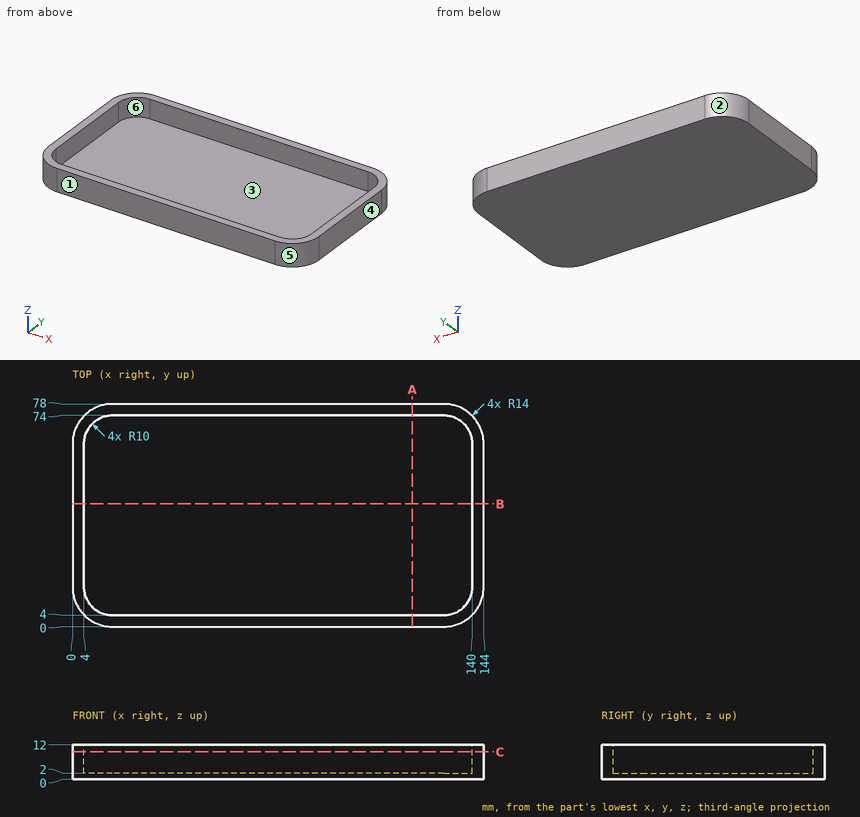
Geometry check sheet. Reference: drawing and pictorial views, mm from the part's lowest x, y, z. A direction names the side the tool comes from. Coordinates: 2 decimals unless noted, no trailing zeros. Write each loop counter-clockwise with the first axis right and the second up, starting at its lowest first coordinate (ties: lowest second). Pieces come first, ordered by that corner, then holes.
Item 1: Depth check by flat-ended pin: pin 1 Ø1 at (x, y) = (117, 37.5) entering from +Z. Enter the tip coordinate at first touch or a pass-through.
Numbers:
pin 1: stops at z = 2
Item 2: Scan lines: probe 1 along Y at (x, z) = (126.5, 3.75); probe 2 along X at (y, z) = (48, 11.25); probe 3 along Z at (x, y) = (51.5, 39.5). Record each from-to range of solid material in increasing order.
Numbers:
probe 1: y = 0 to 4, 74 to 78
probe 2: x = 0 to 4, 140 to 144
probe 3: z = 0 to 2
Item 3: Cross-section at C-C on z = 9.5. Record the boundary of the cut face in (x, y), then the cut area to 3 significant figures.
Numbers:
outline: (0, 14) arc R14 ccw to (14, 0) - (130, 0) arc R14 ccw to (144, 14) - (144, 64) arc R14 ccw to (130, 78) - (14, 78) arc R14 ccw to (0, 64) - close; hole (4, 14) arc R10 ccw to (14, 4) - (130, 4) arc R10 ccw to (140, 14) - (140, 64) arc R10 ccw to (130, 74) - (14, 74) arc R10 ccw to (4, 64) - close
area: 1,630 mm2
Item 4: Mould release check, pull along X, two halves, no side actions. Record for the marked faces 1, 2, 3 and 4: released by +X, released by -X, zero draft, split by the parting line, or undercut.
Numbers:
face 1: zero draft
face 2: released by -X
face 3: undercut
face 4: released by +X
Item 5: Cross-section at A-A on x = 119. Record the boundary of the cut face in (y, z).
Numbers:
outline: (0, 0) - (78, 0) - (78, 12) - (74, 12) - (74, 2) - (4, 2) - (4, 12) - (0, 12) - close
Item 6: Access from +Z, -Z, +X, -X, +Y, -Y to the whole of each face (thin tool, end or side, straight path). Record for the marked faces 5 and 6.
Numbers:
face 5: +Z, -Z, +X, -Y
face 6: +Z
Item 7: Cross-section at B-B on y = 43. Record the boundary of the cut face in (x, z).
Numbers:
outline: (0, 0) - (144, 0) - (144, 12) - (140, 12) - (140, 2) - (4, 2) - (4, 12) - (0, 12) - close
